```python
from build123d import *

# Parameters (mm, degrees)
F2_W      = 14.063794
F2_H      = 1.89093
F2_H_2    = 2.54
F4_R      = 8.89
F5_DEPTH  = 5.334
F6_R      = 8.003634
F6_R_2    = 5.807909
F7_DEPTH  = 7.62
F8_R      = 3.79686
F9_DEPTH  = 25.4
F10_DEPTH = 98.552
F11_R     = 3.354898
F12_DEPTH = 25.4
F13_DEPTH = 156.972


with BuildPart() as f1:
    # F0 (on Front) → F1 (revolve)
    with BuildSketch(Plane.XZ):
        with BuildLine():
            Line((0, 36.400415), (0, 0))
            Line((0, 0), (10.754668, 0))
            ThreePointArc((10.754668, 0), (5.545952, 17.846443), (4.372776, 36.400415))
            Line((4.372776, 36.400415), (0, 36.400415))
        make_face()
    revolve(axis=Axis((0, 0, 22.225), (0, 0, 1)))

    # F2 (on Front) → F3 (revolve)
    with BuildSketch(Plane.XZ):
        Polygon((10.754665, 0), (0, 0), (0, -4.018228), (14.063794, -4.018228), align=None)
        with Locations((7.031897, -4.963693)):
            Rectangle(F2_W, F2_H)
        with Locations((7.031897, -7.179158)):
            Rectangle(F2_W, F2_H_2)
    revolve(axis=Axis((0, 0, -4.963693), (0, 0, 1)))

    # F4 (on face) → F5 (join)
    with BuildSketch(Plane.XY.offset(36.400415)):
        Circle(F4_R)
    extrude(amount=F5_DEPTH)

    # F6 (on face) → F7 (join)
    with BuildSketch(Plane.XY.offset(41.734415)):
        Circle(F6_R)
        Circle(F6_R_2, mode=Mode.SUBTRACT)
    extrude(amount=F7_DEPTH)

    # F8 (on Front) → F9 (cut)
    with BuildSketch(Plane.XZ):
        with Locations((0, 48.400268)):
            Circle(F8_R)
    extrude(amount=-F9_DEPTH, mode=Mode.SUBTRACT)

    # F8 (on Front) → F10 (cut)
    with BuildSketch(Plane.XZ):
        with Locations((0, 48.400268)):
            Circle(F8_R)
    extrude(amount=F10_DEPTH, mode=Mode.SUBTRACT)

    # F11 (on Right) → F12 (cut)
    with BuildSketch(Plane.YZ):
        with Locations((0, 47.958534)):
            Circle(F11_R)
    extrude(amount=-F12_DEPTH, mode=Mode.SUBTRACT)

    # F11 (on Right) → F13 (cut)
    with BuildSketch(Plane.YZ):
        with Locations((0, 47.958534)):
            Circle(F11_R)
    extrude(amount=F13_DEPTH, mode=Mode.SUBTRACT)


solid = f1.part
```
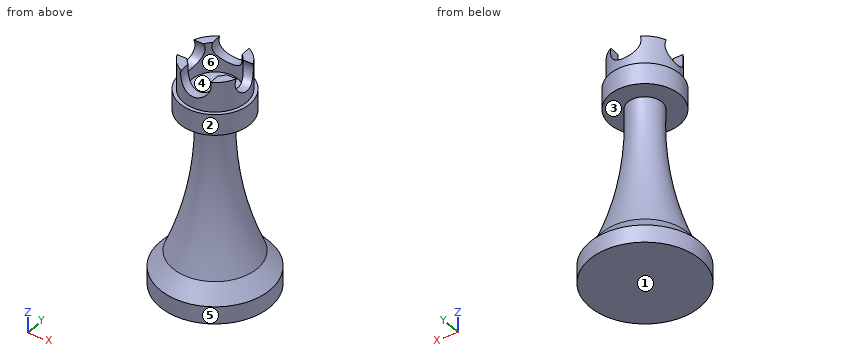
Can you work these out from the model? Positions are in its coordinate system, mm. Face numbers are marked on the shaded views. A direction names the side the tool comes from. Give positions to 0.01 mm unless a question says otherwise; leave off trailing zeros. Order: outer loops, then holes, each group sorted by start corner. A loop starts at its lowest first (then second) coordinate and runs counter-clockwise, first axis right, second up. Notation, with made-up numbers: (-2, 63.25) - (39, 63.25) arc R11 cw to (39, 82.25) - close; hole circle Ø1 at (85.5, 10.5). An arc over 180 degrees is marked (long way). Use a Markdown table: item, result. Add a question column.
Q1. I'm going to push flat-ended pins straight in: pin 1 (4 mm diameter, centred on y = 0, z = 47.96, fed in from +X); pin 2 (3.5 mm diameter, centred on x = -2.5, y = -3, fed in from +Z); pin 3 (10 mm diameter, centred on x = 10, z = 40.5, fed in from -Y); pin 4 (4 mm diameter, centred on x = -0.5, z = 10, fed in from -Y). Where does each tip first touch, or does it pass through?
Q2. Please list where these lines run through material, in increasing order: line 1 along Y through (x, z) = (4.5, 46); line 2 along X through (y, z) = (-4.25, -1); line 3 along X through (y, z) = (3, 26.5).
Q3. If we section it at A-A on z = 44: Write out the boundary of the cut face in (x, y), plus the area to 3 significant figures.
Q4. If we mould it in two halves opening along Z, with no side actions, what happens to the marked faces 1, 2, 3 and 4? For each: released by +Z, released by -Z, zero draft, split by the parting line, or undercut.
Q5. If we section it at D-D on z = -2.5: Write out the boundary of the cut face in (x, y).
Q6. On a 3-axis mill with a long thin cutter (end or side, diameter ignored), from which of +Z, -Z, +X, -X, +Y, -Y can I reach the whole of each face in a straight line? I mean the marked faces 5 and 6. Say none if no direction works.
Answers follow:
| question | item | result |
|---|---|---|
| 1 | pin 1 | passes through |
| 1 | pin 2 | stops at z = 41.73 |
| 1 | pin 3 | stops at y = -7.35 |
| 1 | pin 4 | stops at y = -7.88 |
| 2 | line 1 | y = -6.62 to -3.67, 3.67 to 6.62 |
| 2 | line 2 | x = -10.77 to 10.77 |
| 2 | line 3 | x = -3.34 to 3.34 |
| 3 | outline | circle Ø16.01 at (0, 0); hole circle Ø11.62 at (0, 0) |
| 3 | area | 95.3 mm^2 |
| 4 | face 1 | released by -Z |
| 4 | face 2 | zero draft |
| 4 | face 3 | undercut |
| 4 | face 4 | released by +Z |
| 5 | outline | circle Ø25.63 at (0, 0) |
| 6 | face 5 | +Z, -Z |
| 6 | face 6 | +Z |
